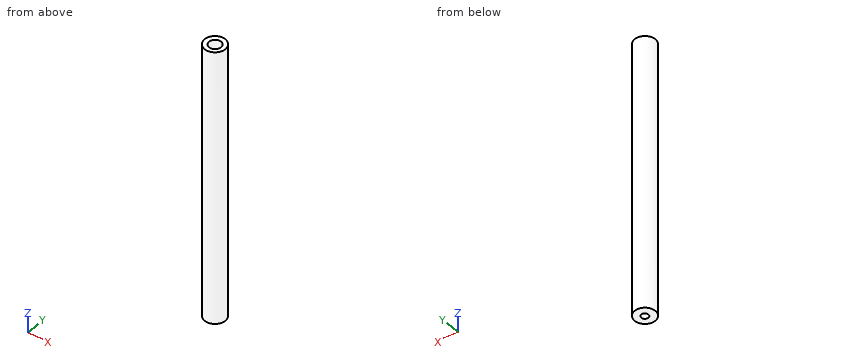
```python
from build123d import *

# Parameters (mm, degrees)
F0_R     = 0.75
F1_DEPTH = 20
F2_R     = 0.4313
F3_DEPTH = 3
F4_R     = 0.3556
F5_DEPTH = 7
F6_R     = 0.254
F7_DEPTH = 7
F8_R     = 0.1461
F9_DEPTH = 3


with BuildPart() as f1:
    # F0 (on Top) → F1 (new body)
    with BuildSketch(Plane.XY):
        with Locations((-0.020624, 0.015056)):
            Circle(F0_R)
    extrude(amount=F1_DEPTH)

    # F2 (on face) → F3 (cut)
    with BuildSketch(Plane.XY.offset(20)):
        Circle(F2_R)
    extrude(amount=-F3_DEPTH, mode=Mode.SUBTRACT)

    # F4 (on face) → F5 (cut)
    with BuildSketch(Plane.XY.offset(17)):
        Circle(F4_R)
    extrude(amount=-F5_DEPTH, mode=Mode.SUBTRACT)

    # F6 (on face) → F7 (cut)
    with BuildSketch(Plane(origin=(0, 0, 0), x_dir=(1, 0, 0), z_dir=(0, 0, -1))):
        Circle(F6_R)
    extrude(amount=-F7_DEPTH, mode=Mode.SUBTRACT)

    # F8 (on face) → F9 (cut)
    with BuildSketch(Plane(origin=(0, 0, 7), x_dir=(1, 0, 0), z_dir=(0, 0, -1))):
        Circle(F8_R)
    extrude(amount=-F9_DEPTH, mode=Mode.SUBTRACT)


solid = f1.part
```
CAD build for the part. Positions are in the model's coordinates, mm. Give positions to 0.01 mm unless a question says otherwise; leave off trailing zeros. Loops run counter-clockwise (first coordinate to the right, second up) from the corner with the lowest first, then second, coordinate; pieces in that order, holes last. Notation, with made-up numbers: (-13, -5) -> (35, -5) arc R10 ccw to (35, 2) -> close; hole circle Ø7 at (67.25, 25.25). An arc over 180 degrees is marked (long way). Use a Markdown table: item, result.
1. Slice it at A-A (z = 5). List the corners of the cut face in (x, y).
Check result:
| item | result |
|---|---|
| outline | circle Ø1.5 at (-0.02, 0.02); hole circle Ø0.51 at (0, 0) |
2. Wall check: L1, parallel to Y at x = 0, z = 18.5; L2, parallel to Y at x = 0, z = 4.5; L3, parallel to X at y = 0, z = 4.75. Give the ranges that are in metal, low to high. Write a range as [from, to].
Check result:
| item | result |
|---|---|
| L1 | y = [-0.73, -0.43], [0.43, 0.76] |
| L2 | y = [-0.73, -0.25], [0.25, 0.76] |
| L3 | x = [-0.77, -0.25], [0.25, 0.73] |
3. Slice it at B-B (z = 13.5). List the corners of the cut face in (x, y), plus the area to 3 significant figures.
Check result:
| item | result |
|---|---|
| outline | circle Ø1.5 at (-0.02, 0.02); hole circle Ø0.71 at (0, 0) |
| area | 1.37 mm^2 |
